For this review, take the finished solid that the model builds, in its own axes (mm). A direction names the side the tool comes from. Coordinates: 2 decimals unless noted, no trailing zeros. Loops run counter-clockwise (first coordinate to the right, second up) from the corner with the lowest first, then second, coordinate; pieces in that order, holes last. Notation, with made-up numbers: (45, 89.5) - (104, 89.5) arc R32 cw to (104, 118.5) - close; hole circle Ø8 at (64.25, 88.25). An arc over 180 degrees is marked (long way). Answer as a JSON object with one key per item and string values. Group by question number.
Item 1: Mouldability with a two-part tool opening along Y and no side actions: class faces 1 (the flat face through (26, -42, 25)), 2 (the flat face through (54, -1, 21)), 3 (the flat face through (2, 45.775, 21)), 4 (the flat face through (26, 0, 2)) as released by +Y, released by -Y, zero draft, split by the parting line, or undercut.
Item 2: Clearance check with a flat-ended pin moving along its axis: pin 1 (4 mm diameter, centred on x = 10.5, y = 22, fed in from +Z). State where the tip first meets the part, or that it passes through.
Item 3: To check wall thickness, follow line 1 (X direction, y = -38.5, z = 4); line 2 (Y direction, x = 17, z = 35) (3 decimals); line 3 (Y direction, x = -20.5, z = 38) (3 decimals). State the ranges of each line that lie inside material, in increasing order.
Item 4: We need section B-B (x = -9.5). Give the boundary of the cut face in (y, z) (3 decimals).
Item 5: We need section D-D (x = 27). Give the boundary of the cut face in (y, z) (3 decimals), then the cut area to 3 significant figures.
Item 6: We need section C-C (y = 32). Give the boundary of the cut face in (x, z), then the cut area to 3 significant figures.
Item 7: We need section A-A (z = 16). Give the boundary of the cut face in (x, y) (3 decimals), then the cut area to 3 significant figures.
Item 8: Tool access review of faces 5 (the flat face through (-48, -1, 21)), 6 (the cylindrical face through (26.2, 39.9, 4)): name each direction out of +Z, -Z, +X, -X, +Y, -Y from which nothing blocks a thin tool from reaching the whole face with its end or side.
from build123d import *

# Parameters (mm, degrees)
F0_W     = 102
F0_H     = 91.55
F0_W_2   = 45
F0_H_2   = 87.55
F0_W_3   = 51
F0_H_3   = 84
F1_DEPTH = 2
F2_DEPTH = 42
F3_R     = 7
F4_R     = 5
F5_R     = 2
F6_SIZE  = 0.5
F7_R     = 1
F8_SIZE  = 0.5


with BuildPart() as f1:
    # F0 (on Top) → F1 (new body)
    with BuildSketch(Plane.XY):
        with Locations((3, 0)):
            Rectangle(F0_W, F0_H)
        with Locations((-23.5, 0)):
            Rectangle(F0_W_2, F0_H_2, mode=Mode.SUBTRACT)
        with Locations((26.5, 0)):
            Rectangle(F0_W_3, F0_H_3, mode=Mode.SUBTRACT)
        with Locations((-23.5, 0)):
            Rectangle(F0_W_2, F0_H_2)
        with Locations((26.5, 0)):
            Rectangle(F0_W_3, F0_H_3)
    extrude(amount=F1_DEPTH)

    # F0 (on Top) → F2 (join)
    with BuildSketch(Plane.XY):
        with Locations((3, 0)):
            Rectangle(F0_W, F0_H)
        with Locations((-23.5, 0)):
            Rectangle(F0_W_2, F0_H_2, mode=Mode.SUBTRACT)
        with Locations((26.5, 0)):
            Rectangle(F0_W_3, F0_H_3, mode=Mode.SUBTRACT)
    extrude(amount=F2_DEPTH)

    # F3
    f3_edges = [f1.edges().sort_by_distance(p)[0] for p in [
        (26.5, 42, 2),
        (26.5, -42, 2),
    ]]
    fillet(f3_edges, radius=F3_R)

    # F4
    f4_edges = [f1.edges().sort_by_distance(p)[0] for p in [
        (-23.5, 43.775, 2),
        (-23.5, -43.775, 2),
    ]]
    fillet(f4_edges, radius=F4_R)

    # F5
    f5_edges = [f1.edges().sort_by_distance(p)[0] for p in [
        (54, -45.775, 21),
        (54, 45.775, 21),
        (-48, 45.775, 21),
        (-48, -45.775, 21),
    ]]
    fillet(f5_edges, radius=F5_R)

    # F6
    f6_edges = [f1.edges().sort_by_distance(p)[0] for p in [
        (-48, 0, 0),
        (-47.414214, 45.189214, 0),
        (-47.414214, -45.189214, 0),
        (3, 45.775, 0),
        (3, -45.775, 0),
        (53.414214, 45.189214, 0),
        (53.414214, -45.189214, 0),
        (54, 0, 0),
    ]]
    chamfer(f6_edges, length=F6_SIZE)

    # F7
    f7_edges = [f1.edges().sort_by_distance(p)[0] for p in [
        (-46, 43.775, 24.5),
        (-1, 0, 2),
        (1, -42, 25.5),
        (52, 42, 25.5),
    ]]
    fillet(f7_edges, radius=F7_R)

    # F8
    f8_edges = [f1.edges().sort_by_distance(p)[0] for p in [
        (-46, 0, 42),
        (-45.707107, -43.482107, 42),
        (-45.707107, 43.482107, 42),
        (-23.5, -43.775, 42),
        (-23.5, 43.775, 42),
        (-1.292893, -43.482107, 42),
        (-1.292893, 43.482107, 42),
        (-1, 0, 42),
        (-48, 0, 42),
        (-47.414214, 45.189214, 42),
        (-47.414214, -45.189214, 42),
        (3, 45.775, 42),
        (3, -45.775, 42),
        (53.414214, 45.189214, 42),
        (53.414214, -45.189214, 42),
        (54, 0, 42),
        (26.5, -42, 42),
        (51.707107, -41.707107, 42),
        (1.292893, -41.707107, 42),
        (52, 0, 42),
        (1, 0, 42),
        (51.707107, 41.707107, 42),
        (1.292893, 41.707107, 42),
        (26.5, 42, 42),
    ]]
    chamfer(f8_edges, length=F8_SIZE)


solid = f1.part
Check sheet entries:
{
 "1": {"face 1": "undercut", "face 2": "zero draft", "face 3": "released by +Y", "face 4": "undercut"},
 "2": {"pin 1": "stops at z = 2"},
 "3": {"line 1": "x = -48 to -46, -1 to 1.01, 51.99 to 54", "line 2": "y = -45.775 to -42, 42 to 45.775", "line 3": "y = -45.775 to -43.775, 43.775 to 45.775"},
 "4": {"outline": "(-45.775, 0.5) - (-45.275, 0) - (45.275, 0) - (45.775, 0.5) - (45.775, 41.5) - (45.275, 42) - (44.275, 42) - (43.775, 41.5) - (43.775, 7) arc R5 cw to (38.775, 2) - (-38.775, 2) arc R5 cw to (-43.775, 7) - (-43.775, 41.5) - (-44.275, 42) - (-45.275, 42) - (-45.775, 41.5) - close"},
 "5": {"outline": "(-45.775, 0.5) - (-45.275, 0) - (45.275, 0) - (45.775, 0.5) - (45.775, 41.5) - (45.275, 42) - (42.5, 42) - (42, 41.5) - (42, 9) arc R7 cw to (35, 2) - (-35, 2) arc R7 cw to (-42, 9) - (-42, 41.5) - (-42.5, 42) - (-45.275, 42) - (-45.775, 41.5) - close", "area": "505 mm2"},
 "6": {"outline": "(-48, 0.5) - (-47.5, 0) - (53.5, 0) - (54, 0.5) - (54, 41.5) - (53.5, 42) - (52.5, 42) - (52, 41.5) - (52, 3) arc R1 cw to (51, 2) - (2, 2) arc R1 cw to (1, 3) - (1, 41.5) - (0.5, 42) - (-0.5, 42) - (-1, 41.5) - (-1, 3) arc R1 cw to (-2, 2) - (-45, 2) arc R1 cw to (-46, 3) - (-46, 41.5) - (-46.5, 42) - (-47.5, 42) - (-48, 41.5) - close", "area": "444 mm2"},
 "7": {"outline": "(-48, -43.775) arc R2 ccw to (-46, -45.775) - (52, -45.775) arc R2 ccw to (54, -43.775) - (54, 43.775) arc R2 ccw to (52, 45.775) - (-46, 45.775) arc R2 ccw to (-48, 43.775) - close; hole (-46, -42.775) arc R1 ccw to (-45, -43.775) - (-2, -43.775) arc R1 ccw to (-1, -42.775) - (-1, 42.775) arc R1 ccw to (-2, 43.775) - (-45, 43.775) arc R1 ccw to (-46, 42.775) - close; hole (1, -41) arc R1 ccw to (2, -42) - (51, -42) arc R1 ccw to (52, -41) - (52, 41) arc R1 ccw to (51, 42) - (2, 42) arc R1 ccw to (1, 41) - close", "area": "1,110 mm2"},
 "8": {"face 5": "+Z, -Z, -X, +Y, -Y", "face 6": "+Z"}
}
